Work out the finished part from the listing and answer in its coordinate system (mm). A direction names the side the tool comes from. Coordinates: 2 decimals unless noted, no trailing zeros. Order: outer loops, then holes, each group sorted by start corner. A loop starts at its lowest first (then second) coordinate and runs counter-clockwise, first axis right, second up.
```python
from build123d import *

# Parameters (mm, degrees)
SKETCH1_W           = 101.6
SKETCH1_H           = 25.4
BOSS_EXTRUDE1_DEPTH = 215.9
SKETCH3_R           = 5.207
CUT_EXTRUDE1_DEPTH  = 17.78
SKETCH4_R           = 4.953
BOSS_EXTRUDE3_DEPTH = 17.78
SKETCH8_W           = 101.6
SKETCH8_H           = 215.9
BOSS_EXTRUDE4_DEPTH = 34
CUT_EXTRUDE2_DEPTH  = 217
SKETCH14_R          = 3.5
CUT_EXTRUDE3_DEPTH  = 9
FILLET1_R           = 5
FILLET2_R           = 5
SKETCH16_W          = 24.7
SKETCH16_H          = 96
CUT_EXTRUDE4_DEPTH  = 42
SKETCH17_W          = 24.7
SKETCH17_H          = 96
CUT_EXTRUDE5_DEPTH  = 42


with BuildPart() as part:
    # Sketch1 → Boss-Extrude1 (new body)
    with BuildSketch(Plane(origin=(0, 0, 0), x_dir=(1, 0, 0), z_dir=(0, 1, 0))):
        with Locations((25.4, 12.7)):
            Rectangle(SKETCH1_W, SKETCH1_H)
    extrude(amount=BOSS_EXTRUDE1_DEPTH)

    # Sketch3 → Cut-Extrude1 (cut)
    with BuildSketch(Plane(origin=(0, 0, 0), x_dir=(-1, 0, 0), z_dir=(0, -1, 0))):
        with Locations(Location((5.08, 12.7, 0), (0, 0, 90))):
            Circle(SKETCH3_R)
        with Locations(Location((-55.88, 12.7, 0), (0, 0, 90))):
            Circle(SKETCH3_R)
    extrude(amount=-CUT_EXTRUDE1_DEPTH, mode=Mode.SUBTRACT)

    # Sketch4 → Boss-Extrude3 (add)
    with BuildSketch(Plane(origin=(0, 215.9, 0), x_dir=(1, 0, 0), z_dir=(0, 1, 0))):
        with Locations(Location((-5.08, 12.7, 0), (0, 0, 270))):
            Circle(SKETCH4_R)
        with Locations(Location((55.88, 12.7, 0), (0, 0, 270))):
            Circle(SKETCH4_R)
    extrude(amount=BOSS_EXTRUDE3_DEPTH)

    # Sketch8 → Boss-Extrude4 (add)
    with BuildSketch(Plane(origin=(0, 0, -25.4), x_dir=(-1, 0, 0), z_dir=(0, 0, -1))):
        with Locations((-25.4, 107.95)):
            Rectangle(SKETCH8_W, SKETCH8_H)
    extrude(amount=BOSS_EXTRUDE4_DEPTH)

    # Sketch10 → Cut-Extrude2 (cut)
    with BuildSketch(Plane(origin=(0, 215.9, 0), x_dir=(1, 0, 0), z_dir=(0, 1, 0))):
        Polygon((-25.4, 54.4), (-5.4, 54.4), (-25.4, 29.7), align=None)
        Polygon((76.2, 54.4), (56.2, 54.4), (76.2, 29.7), align=None)
    extrude(amount=-CUT_EXTRUDE2_DEPTH, mode=Mode.SUBTRACT)

    # Sketch14 → Cut-Extrude3 (cut)
    with BuildSketch(Plane(origin=(0, 0, -59.4), x_dir=(-1, 0, 0), z_dir=(0, 0, -1))):
        with Locations((-41.400000283, 129.695762338)):
            Circle(SKETCH14_R)
        with Locations((-9.400000283, 129.695762338)):
            Circle(SKETCH14_R)
        with Locations((-41.400000283, 93.695762338)):
            Circle(SKETCH14_R)
        with Locations((-9.400000283, 93.695762338)):
            Circle(SKETCH14_R)
    extrude(amount=-CUT_EXTRUDE3_DEPTH, mode=Mode.SUBTRACT)

    # Fillet1
    fillet1_edges = [part.edges().sort_by_distance(p)[0] for p in [
        (-25.4, 107.95, 0),
    ]]
    fillet(fillet1_edges, radius=FILLET1_R)

    # Fillet2
    fillet2_edges = [part.edges().sort_by_distance(p)[0] for p in [
        (76.2, 107.95, 0),
    ]]
    fillet(fillet2_edges, radius=FILLET2_R)

    # Sketch16 → Cut-Extrude4 (cut)
    with BuildSketch(Plane.ZY.offset(25.4)):
        with Locations((-42.05, 110.012919034)):
            Rectangle(SKETCH16_W, SKETCH16_H)
    extrude(amount=-CUT_EXTRUDE4_DEPTH, mode=Mode.SUBTRACT)

    # Sketch17 → Cut-Extrude5 (cut)
    with BuildSketch(Plane(origin=(76.2, 0, 0), x_dir=(0, 0, -1), z_dir=(1, 0, 0))):
        with Locations((42.05, 107.199291506)):
            Rectangle(SKETCH17_W, SKETCH17_H)
    extrude(amount=-CUT_EXTRUDE5_DEPTH, mode=Mode.SUBTRACT)


solid = part.part
```
1. The part is cut by section C-C (y = 168.5). Determine the outline of the cut face in (x, z), plus the area to 3 significant figures.
2. The part is cut by section B-B (z = -12.7). Determine the outline of the cut face in (x, y), plus the area to 3 significant figures.
3. Flat-ended cylindrical pins translate along their axes: pin 1 (2 mm diameter, centred on y = 202, z = -39.5, fed in from -X); pin 2 (5 mm diameter, centred on x = -5.5, z = -11, fed in from -Y); pin 3 (12.5 mm diameter, centred on y = 118.5, z = -37, fed in from -X). Find the tip coordinate at first contact, or state that the pin passes through.
4. The part is cut by section D-D (x = 25). Determine the outline of the cut face in (y, z), plus the area to 3 significant figures.
5. The mould has two halves that part along Y. Classify faces 6 (the flat face through (-9, 109, -54.4)), 7 (the cylindrical face through (-23.9, 109.46, -1.43)): released by +Y, released by -Y, zero draft, split by the parting line, or undercut.
6. For faces 1 (the cylindrical face through (-3.516, 8.766, -17.667)), 2 (the flat face through (0, 158.013, -42)), 3 (the cylindrical face through (41.856, 133.166, -56.935)), 4 (the cylindrical face through (60.06, 224.67, -10.04)), 5 (the flat face through (51, 59.199, -42)), determine the directions among +Z, -Z, +X, -X, +Y, -Y from which every point of the face is accessible in a straight line to the end or side of a thin tool.
7. Consider probe 1 along Y at (x, z) = (9, -56); probe 2 along X at (y, z) = (9.75, -12.7); probe 3 along Z at (x, y) = (-13.5, 63). Determine where each line is inside the solid, lowest interval first.
8. The part is cut by section A-A (x = 9.4). Determine the outline of the cut face in (y, z).
Worked out:
1. outline: (-25.4, -59.4) - (76.2, -59.4) - (76.2, -54.4) - (56.2, -54.4) - (76.2, -29.7) - (76.2, -5) arc R5 ccw to (71.2, 0) - (-20.4, 0) arc R5 ccw to (-25.4, -5) - (-25.4, -29.7) - (-5.4, -54.4) - (-25.4, -54.4) - close
1. area: 5,530 mm2
2. outline: (-25.4, 0) - (-10.29, 0) - (-10.29, 17.78) - (0.13, 17.78) - (0.13, 0) - (50.67, 0) - (50.67, 17.78) - (61.09, 17.78) - (61.09, 0) - (76.2, 0) - (76.2, 215.9) - (60.83, 215.9) - (60.83, 233.68) - (50.93, 233.68) - (50.93, 215.9) - (-0.13, 215.9) - (-0.13, 233.68) - (-10.03, 233.68) - (-10.03, 215.9) - (-25.4, 215.9) - close
2. area: 21,900 mm2
3. pin 1: stops at x = -18.27
3. pin 2: stops at y = 17.78
3. pin 3: stops at x = 16.6
4. outline: (0, -59.4) - (215.9, -59.4) - (215.9, 0) - (0, 0) - close
4. area: 12,800 mm2
5. face 6: undercut
5. face 7: zero draft
6. face 1: -Y
6. face 2: -X
6. face 3: -Z
6. face 4: +Y
6. face 5: +X
7. probe 1: y = 0 to 90.22, 97.17 to 126.22, 133.17 to 215.9
7. probe 2: x = -25.4 to -10.29, 0.13 to 50.67, 61.09 to 76.2
7. probe 3: z = -59.4 to -54.4, -29.7 to 0
8. outline: (0, -59.4) - (90.2, -59.4) - (90.2, -54.4) - (62.01, -54.4) - (62.01, -29.7) - (158.01, -29.7) - (158.01, -54.4) - (133.2, -54.4) - (133.2, -59.4) - (215.9, -59.4) - (215.9, 0) - (0, 0) - close; (97.2, -59.4) - (126.2, -59.4) - (126.2, -54.4) - (97.2, -54.4) - close
